Build history of the part. All positions in model axes, mm. Round coordinates to 2 decimals unless told otherwise and drop trailing zeros. Write each loop counter-clockwise with the first axis right and the second up, starting at its lowest first coordinate (ties: lowest second). Pieces come first, ordered by that corner, then holes. Notation, with made-up numbers: M 14,-30.5 L 28,-30.5 A17 cw 28,-10.5 Z; hole C 16,23 d2. An arc over 180 degrees is marked long. Write item = value, one per line.
from build123d import *


with BuildPart() as f1:
    # F0 (on Front) → F1 (revolve)
    with BuildSketch(Plane.XZ):
        Polygon((0, 32.483602), (0, 0), (0, -32.483602), (5, -32.483602), (5, -30.483602), (2.5, -30.483602), (1.5, 0), (2.5, 30.483602), (5, 30.483602), (5, 32.483602), align=None)
        with BuildLine():
            Line((5, -32.483602), (0, -32.483602))
            Line((0, -32.483602), (0, -37.483602))
            ThreePointArc((0, -37.483602), (3.535534, -36.019136), (5, -32.483602))
        make_face()
        with BuildLine():
            Line((0, 37.483602), (0, 32.483602))
            Line((0, 32.483602), (5, 32.483602))
            ThreePointArc((5, 32.483602), (3.535534, 36.019136), (0, 37.483602))
        make_face()
    revolve(axis=Axis((0, 0, 16.241801), (0, 0, 1)))


solid = f1.part
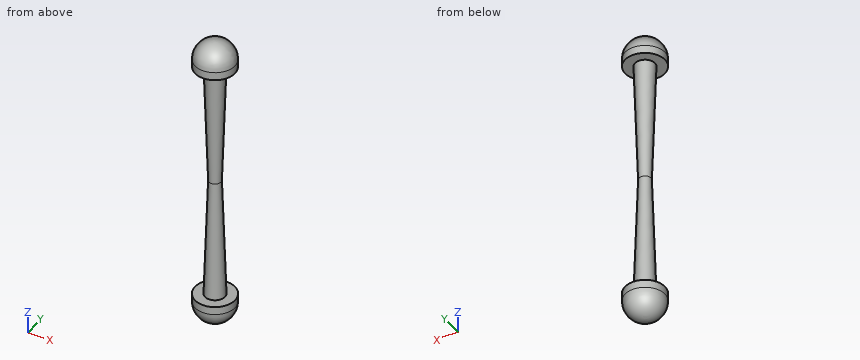
1. Band-saw the part on A-A (z = 16). List the corners of the cut face in (x, y).
Responses:
outline = C 0,0 d4.05
2. Flat gauge pins, fed straight in: pin 1 (4 mm diameter, centred on x = 2, y = -0.5, fed in from +Z); pin 2 (6 mm diameter, centred on y = -2, z = -6, fed in from -X); pin 3 (2 mm diameter, centred on y = -2.5, z = -20.5, fed in from +X); pin 4 (2 mm diameter, centred on x = -2, z = -25.5, fed in from +Y). Where does each tip first touch, or does it go through?
Responses:
pin_1 = 37.48
pin_2 = -1.77
pin_3 = 1.57
pin_4 = 2.11
3. Probe probe 1 along Z at (x, y) = (-0.25, 3.75); probe 2 along Z at (x, y) = (-1.75, -2.75); probe 3 along Y at (x, z) = (-1.25, 1). List the from-to ranges inside material, lowest first.
Responses:
probe_1 = -35.78 to -30.48, 30.48 to 35.78
probe_2 = -36.28 to -30.48, 30.48 to 36.28
probe_3 = -0.89 to 0.89
4. Band-saw the part on B-B (z = 24). List the corners of the cut face in (x, y), plus the area to 3 significant figures.
Responses:
outline = C 0,0 d4.57
area = 16.4 mm²
